Part model, mm, in its own coordinate system. Face numbers are marked on the shaded views. Coordinates: 2 decimals unless noted, no trailing zeros. Loops run counter-clockwise (first coordinate to the right, second up) from the corner with the lowest first, then second, coordinate; pieces in that order, holes last. Notation, with made-up numbers: (-4.5, 14) -> (10.5, 14) arc R6 cw to (10.5, 21) -> close; hole circle Ø4 at (7, -29.5). An arc over 180 degrees is marked (long way). Use one line per item in the form item = value. Start each with the question number.
(1) Band-saw the part on A-A on y = -44.45. Give the cut face in (x, z).
(2) Pin check, flat tips, straight feed: P1, Ø3, axis at x = -11.5, z = 22, coming from the -Y side; P2, Ø12, axis at x = 13, z = -5, coming from the +Y side; P3, Ø3, axis at x = 9.5, y = -29.5, coming from the +Z side. Stop position of each tip, or through.
(3) Band-saw the part on B-B on y = -56. Give the cut face in (x, z), then the cut area to 3 significant figures.
(4) Mould opens along Z. For the marked faces 1 and 2 say: +Z half, -Z half, draft (parallel to the pull), parting line (faces both ways), or undercut.
(5) Drill centre lines: L1, parallel to Y at x = 0, z = 34.15; L2, parallel to Y at x = -29, z = 21 (3 decimals); L3, parallel to Z at x = 0, y = -33.5. Where is each one in solid material? Low to high. Write a range as [from, to].
(6) Band-saw the part on C-C on x = 24. Count the separate pieces of the cut face and the enclosed holes in it, then the cut area to 3 significant figures.
```python
from build123d import *

# Parameters (mm, degrees)
F_19_0_164_DIAMETER_HOLE1_D = 4.1656
CIRPATTERN2_COUNT           = 6


with BuildPart() as part:
    # Sketch1 → Revolve2 (revolve)
    with BuildSketch(Plane.XY):
        with BuildLine():
            Line((0, -25.4), (33.2105, -25.4))
            Line((33.2105, -25.4), (33.2105, -63.5))
            Line((33.2105, -63.5), (36.3855, -63.5))
            Line((36.3855, -63.5), (36.3855, -6.985))
            Line((36.3855, -6.985), (35.1409, -6.985))
            Line((35.1409, -6.985), (35.1409, -4.572))
            Line((35.1409, -4.572), (36.3855, -4.572))
            Line((36.3855, -4.572), (36.3855, 0))
            Line((36.3855, 0), (33.2105, 0))
            ThreePointArc((33.2105, 0), (16.798390624, -3.802656831), (0, -5.08))
            Line((0, -5.08), (0, -25.4))
        make_face()
    revolve(axis=Axis((0, 0, 0), (0, -1, 0)))

    # #19 (0.164) Diameter Hole1 (through all)
    with Locations(Plane(origin=(0, -19.049997805, 36.3855), x_dir=(1, 0, 0), z_dir=(0, 0, 1))):
        with Locations((0, 0), (0, -25.400002195)):
            f_19_0_164_diameter_hole1 = Hole(F_19_0_164_DIAMETER_HOLE1_D / 2)

    # CirPattern2: #19 (0.164) Diameter Hole1 ×6 about axis
    cirpattern2_axis = Axis((0, 0, 0), (0, -1, 0))
    for i in range(1, CIRPATTERN2_COUNT):
        add(f_19_0_164_diameter_hole1.rotate(cirpattern2_axis, i * 360 / CIRPATTERN2_COUNT), mode=Mode.SUBTRACT)


solid = part.part
```
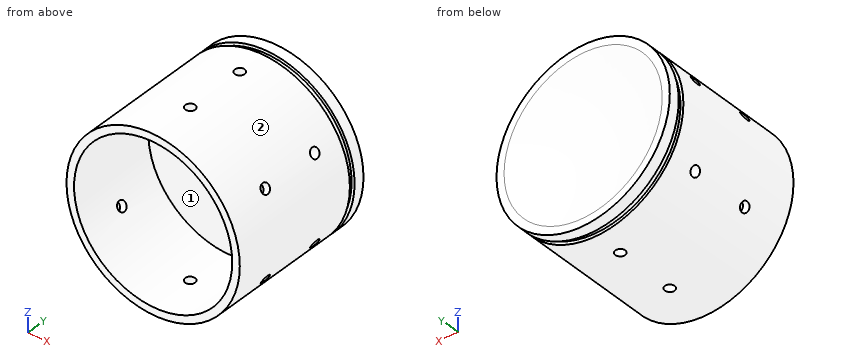
A:
q1.outline = (-32.5, -16.36) -> (-29.75, -14.77) arc R33.21 cw to (-29.75, 14.77) -> (-32.5, 16.36) arc R36.39 ccw to start; (-30.42, -19.97) arc R36.39 ccw to (-2.08, -36.33) -> (-2.08, -33.15) arc R33.21 cw to (-27.66, -18.38) -> close; (-30.42, 19.97) -> (-27.66, 18.38) arc R33.21 cw to (-2.08, 33.15) -> (-2.08, 36.33) arc R36.39 ccw to start; (2.08, -36.33) arc R36.39 ccw to (30.42, -19.97) -> (27.66, -18.38) arc R33.21 cw to (2.08, -33.15) -> close; (2.08, 33.15) arc R33.21 cw to (27.66, 18.38) -> (30.42, 19.97) arc R36.39 ccw to (2.08, 36.33) -> close; (29.75, -14.77) -> (32.5, -16.36) arc R36.39 ccw to (32.5, 16.36) -> (29.75, 14.77) arc R33.21 cw to start
q2.P1 = -25.4
q2.P2 = -3.28
q2.P3 = 35.5
q3.outline = circle Ø72.77 at (0, 0); hole circle Ø66.42 at (0, 0)
q3.area = 694 mm²
q4.face_1 = undercut
q4.face_2 = parting line
q5.L1 = [-63.5, -46.53], [-42.37, -21.13], [-16.97, 0]
q5.L2 = [-63.5, -6.985], [-4.572, 0]
q5.L3 = [-36.39, -33.21], [33.21, 36.39]
q6.separate_pieces = 1
q6.enclosed_holes = 2
q6.area = 1,610 mm²
